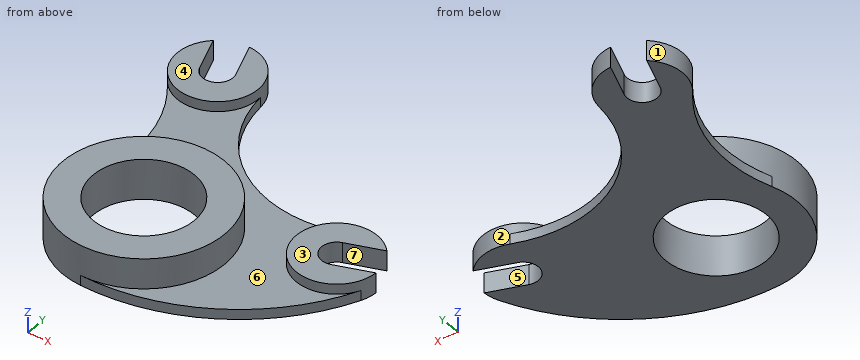
from build123d import *

# Parameters (mm, degrees)
BOSS_EXTRUDE1_DEPTH = 6.35
BOSS_EXTRUDE2_DEPTH = 12.7
SKETCH1_4_R         = 50.8
SKETCH1_4_R_2       = 31.75
BOSS_EXTRUDE3_DEPTH = 25.4


with BuildPart() as part:
    # Sketch1 → Boss-Extrude1 (new body)
    with BuildSketch(Plane.XY):
        with BuildLine():
            ThreePointArc((72.649235075, 31.372352915), (4.684377865, 37.027544064), (-31.532761281, 94.816140123))
            ThreePointArc((-31.532761281, 94.816140123), (-47.103439421, 68.915388021), (-76.423524765, 76.238472936))
            ThreePointArc((-76.423524765, 76.238472936), (-57.493211559, 35.124721846), (-61.259500498, -9.980847149))
            ThreePointArc((-61.259500498, -9.980847149), (-4.767373791, 23.108705876), (37.42041065, -26.955949752))
            ThreePointArc((37.42041065, -26.955949752), (21.901301878, -63.505897962), (-15.174026915, -77.724246886))
            ThreePointArc((-15.174026915, -77.724246886), (56.54324661, -58.54842731), (105.288459403, -2.557502975))
            ThreePointArc((105.288459403, -2.557502975), (63.787892957, -9.815690456), (72.649235075, 31.372352915))
        make_face()
    extrude(amount=BOSS_EXTRUDE1_DEPTH)

    # Sketch1_3 → Boss-Extrude2 (add)
    with BuildSketch(Plane.XY):
        with BuildLine():
            ThreePointArc((-65.766719765, 89.127271222), (-53.558405687, 83.434440874), (-47.865575339, 95.642754953))
            Line((-47.865575339, 95.642754953), (-55.91892877, 117.769161654))
            ThreePointArc((-55.91892877, 117.769161654), (-48.128835912, 68.516820519), (-73.820073196, 111.253677924))
            Line((-73.820073196, 111.253677924), (-65.766719765, 89.127271222))
        make_face()
        with BuildLine():
            ThreePointArc((78.835439057, 16.743869022), (73.142608709, 4.535554944), (85.350922787, -1.157275404))
            Line((85.350922787, -1.157275404), (107.477329489, 6.896078027))
            ThreePointArc((107.477329489, 6.896078027), (58.224988354, -0.894014831), (100.961845758, 24.797222453))
            Line((100.961845758, 24.797222453), (78.835439057, 16.743869022))
        make_face()
    extrude(amount=BOSS_EXTRUDE2_DEPTH)

    # Sketch1_4 → Boss-Extrude3 (add)
    with BuildSketch(Plane.XY):
        with Locations(Location((-13.37958935, -26.955949752, 0), (0, 0, 160.478803641))):
            Circle(SKETCH1_4_R)
        with Locations((-13.37958935, -26.955949752)):
            Circle(SKETCH1_4_R_2, mode=Mode.SUBTRACT)
    extrude(amount=BOSS_EXTRUDE3_DEPTH)


solid = part.part
The listing builds one solid part. Answer for the finished solid, in the listing's coordinates (mm). Face numbers are marked on the shaded views. A direction names the side the tool comes from. Coordinates: 2 decimals unless noted, no trailing zeros. Loops run counter-clockwise (first coordinate to the right, second up) from the corner with the lowest first, then second, coordinate; pieces in that order, holes last. Notation, with made-up numbers: M 77,43 L 114,43 A5 cw 114,49 Z; hole C 31.25,41.5 d7. An arc over 180 degrees is marked long. Answer in a Markdown table with one row per item.
1) Find section B-B (x = 93). Determine the outline of the cut face in (y, z), then the cut area to 3 significant figures.
Answers below:
| item | result |
|---|---|
| outline | M -24.14,0 L 1.63,0 L 1.63,12.7 L -15.15,12.7 L -15.15,6.35 L -24.14,6.35 Z; M 21.9,0 L 30.73,0 L 30.73,12.7 L 21.9,12.7 Z |
| area | 382 mm^2 |
2) Given pin 1 (8 mm diameter, centred on y = 7, z = 13.5, fed in from -X); pin 2 (15 mm diameter, centred on x = -48, y = 102, fed in from +Z); pin 3 (12 mm diameter, centred on x = 29.5, z = 8.5, fed in from +Y), each flat-ended and moving along its own axis, determine where each tip first touches the part or whether it passes through.
Answers below:
| item | result |
|---|---|
| pin 1 | x = -54.41 |
| pin 2 | z = 12.7 |
| pin 3 | y = 28.7 |
3) Determine the mould class of the marked faces 1, 2 and 3 for opening direction Y: released by +Y, released by -Y, zero draft, split by the parting line, or undercut.
Answers below:
| item | result |
|---|---|
| face 1 | undercut |
| face 2 | split by the parting line |
| face 3 | zero draft |
4) Find section A-A (z = 10). Count the separate pieces of the cut face and the enclosed holes in it, then the cut area to 3 significant figures.
Answers below:
| item | result |
|---|---|
| separate pieces | 3 |
| enclosed holes | 1 |
| area | 7,760 mm^2 |
5) Which of the six approach directions +Z, -Z, +X, -X, +Y, -Y give full straight-line access (tool end or side, diameter ignored) to the marked faces 4, 5, 6 and 7?
Answers below:
| item | result |
|---|---|
| face 4 | +Z, +X, -X, +Y |
| face 5 | +Z, -Z |
| face 6 | +Z |
| face 7 | +Z, -Z, +X |
6) Find section D-D (y = -64). Determine the outline of the cut face in (x, z), then the cut area to 3 significant figures.
Answers below:
| item | result |
|---|---|
| outline | M -48.14,0 L 46.89,0 L 46.89,6.35 L 21.38,6.35 L 21.38,25.4 L -48.14,25.4 Z |
| area | 1,930 mm^2 |
7) Find the intervals of material crossed by probe 1 along Y at (x, z) = (-7, 18.5); probe 2 along Y at (x, z) = (-30, 12.5); probe 3 along Z at (x, y) = (-31, 23), in increasing order.
Answers below:
| item | result |
|---|---|
| probe 1 | -77.35 to -58.06, 4.15 to 23.44 |
| probe 2 | -74.96 to -54.01, 0.1 to 21.05 |
| probe 3 | 0 to 6.35 |
8) Find section C-C (y = 100). Determine the outline of the cut face in (x, z), then the cut area to 3 significant figures.
Answers below:
| item | result |
|---|---|
| outline | M -81.05,0 L -69.72,0 L -69.72,12.7 L -81.05,12.7 Z; M -49.45,0 L -32.58,0 L -32.58,12.7 L -49.45,12.7 Z |
| area | 358 mm^2 |
